from build123d import *

# Parameters (mm, degrees)
SKETCH1_R            = 30
BOSS_EXTRUDE1_DEPTH  = 75
SKETCH2_W            = 10
SKETCH2_H            = 56.81
SKETCH2_H_2          = 73.19
SKETCH3_R            = 3.175
BOSS_EXTRUDE2_DEPTH  = 10
SKETCH5_W            = 10
SKETCH5_H            = 20
CUT_EXTRUDE2_DEPTH   = 30
FILLET1_R            = 15
FILLET1_OF_MIRROR1_R = 15


with BuildPart() as part:
    # Sketch1 → Boss-Extrude1 (new, symmetric)
    with BuildSketch(Plane(origin=(0, 0, 0), x_dir=(1, 0, 0), z_dir=(0, 1, 0))):
        with Locations(Location((0, 0, 0), (0, 0, 270))):
            Circle(SKETCH1_R)
    extrude(amount=BOSS_EXTRUDE1_DEPTH, both=True)

    # Sketch2 → Cut-Revolve1 (revolve, cut)
    with BuildSketch(Plane(origin=(0, 0, 0), x_dir=(0, 0, -1), z_dir=(1, 0, 0))):
        with Locations((25, 36.595)):
            Rectangle(SKETCH2_W, SKETCH2_H)
        with Locations((25, -38.405)):
            Rectangle(SKETCH2_W, SKETCH2_H_2)
    revolve(axis=Axis((0, -1000, 0), (0, 1, 0)), mode=Mode.SUBTRACT)

    # Sketch3 → Boss-Extrude2 (add, symmetric)
    with BuildSketch(Plane(origin=(0, 0, 0), x_dir=(0, 0, -1), z_dir=(1, 0, 0))):
        Polygon((0, 75), (0, 60), (70, 60), (70, 85), (50, 85), (50, 75), align=None)
        with Locations((60, 75)):
            Circle(SKETCH3_R, mode=Mode.SUBTRACT)
    boss_extrude2 = extrude(amount=BOSS_EXTRUDE2_DEPTH, both=True)

    # Sketch5 → Cut-Extrude2 (cut)
    with BuildSketch(Plane(origin=(0, 0, -70), x_dir=(-1, 0, 0), z_dir=(0, 0, -1))):
        with Locations((0, 75)):
            Rectangle(SKETCH5_W, SKETCH5_H)
    cut_extrude2 = extrude(amount=-CUT_EXTRUDE2_DEPTH, mode=Mode.SUBTRACT)

    # Fillet1
    # the kernel refuses this fillet: 15 mm, written as the material it takes off along each edge
    with BuildSketch(Plane(origin=(-47.5, 60, -70), x_dir=(0, 0, 1), z_dir=(1, 0, 0))) as fillet1_piece_1:
        with BuildLine():
            CenterArc((FILLET1_R, -FILLET1_R), FILLET1_R, 90, 90)
            Line((0, -FILLET1_R), (0, 0))
            Line((0, 0), (FILLET1_R, 0))
        make_face()
    extrude(amount=95, mode=Mode.SUBTRACT)

    # Mirror1: Boss-Extrude2, Cut-Extrude2 across plane
    add(boss_extrude2.mirror(Plane.XY))
    add(cut_extrude2.mirror(Plane.XY), mode=Mode.SUBTRACT)

    # Fillet1 of Mirror1
    # the kernel refuses this fillet: 15 mm, written as the material it takes off along each edge
    with BuildSketch(Plane(origin=(-47.5, 60, 70), x_dir=(0, 0, -1), z_dir=(1, 0, 0))) as fillet1_of_mirror1_piece_1:
        with BuildLine():
            CenterArc((FILLET1_OF_MIRROR1_R, FILLET1_OF_MIRROR1_R), FILLET1_OF_MIRROR1_R, 180, 90)
            Line((0, FILLET1_OF_MIRROR1_R), (0, 0))
            Line((0, 0), (FILLET1_OF_MIRROR1_R, 0))
        make_face()
    extrude(amount=95, mode=Mode.SUBTRACT)


solid = part.part
Here's how the part is built. I have some questions about the finished solid (model axes, mm). A direction names the side the tool comes from. Round coordinates to 2 decimals unless told otherwise and drop trailing zeros. Order: outer loops, then holes, each group sorted by start corner. A loop starts at its lowest first (then second) coordinate and runs counter-clockwise, first axis right, second up. Notation, with made-up numbers: M -27.5,-24.75 L 14.5,-24.75 A25 cw 14.5,-11.75 Z; hole C 83,31.5 d7. An arc over 180 degrees is marked long. One line per question, with ' | ' between items.
1) I'm going to push flat-ended pins straight in: pin 1 Ø7.5 at (y, z) = (75, 60) entering from +X; pin 2 Ø18 at (x, z) = (-2, -1.5) entering from +Y; pin 3 Ø7.5 at (y, z) = (72, -36) entering from -X. Where does each tip first touch, or does it pass through?
Checked values:
pin 1: stops at x = 10 | pin 2: stops at y = 75 | pin 3: stops at x = -10
2) Imagine slicing it at A-A, the plane x = 0. Write out the boundary of the cut face in (y, z), plus the area to 3 significant figures.
Checked values:
outline: M -75,-20 L -1.81,-20 L -1.81,-30 L 8.19,-30 L 8.19,-20 L 60,-20 L 60,-55 A15 ccw 65,-66.18 L 65,-40 L 75,-40 L 75,40 L 65,40 L 65,66.18 A15 ccw 60,55 L 60,20 L 8.19,20 L 8.19,30 L -1.81,30 L -1.81,20 L -75,20 Z | area: 7,030 mm²
3) On a 3-axis mill with a long thin cutter (end or side, diameter ignored), from which of +Z, -Z, +X, -X, +Y, -Y can I reach the whole of each face in a straight line? I mean faces 4 (the flat face through (0, 75, -1)), 5 (the cylindrical face through (-7.535, 77.677, 61.707)), 6 (the flat face through (-5, 75, -55)), 7 (the flat face through (22, 65, 0)), 8 (the flat face through (20, 8.19, 6)). Say none if no direction works.
Checked values:
face 4: +X, -X, +Y | face 5: +X, -X | face 6: -Z, +Y | face 7: +X | face 8: none
4) Imagine slicing it at D-D, the plane z = -60. Write out the boundary of the cut face in (x, y) (3 decimals), plus the area to 3 significant figures.
Checked values:
outline: M -10,60.858 L 10,60.858 L 10,71.825 L 5,71.825 L 5,65 L -5,65 L -5,71.825 L -10,71.825 Z; M -10,78.175 L -5,78.175 L -5,85 L -10,85 Z; M 5,78.175 L 10,78.175 L 10,85 L 5,85 Z | area: 219 mm²
5) We'd pull the mould along X, two halves only. Please class faces 1 (the flat face through (5, 75, 55)), 2 (the cylindrical face through (19.524, -37.893, 4.336)), 3 (the cylindrical face through (29.996, 70.07, 0.517)): released by +X, released by -X, zero draft, split by the parting line, or undercut.
Checked values:
face 1: undercut | face 2: split by the parting line | face 3: released by +X
6) Imagine slicing it at B-B, the plane z = 0. Write out the boundary of the cut face in (x, y), plus the area to 3 significant figures.
Checked values:
outline: M -30,-1.81 L -20,-1.81 L -20,-75 L 20,-75 L 20,-1.81 L 30,-1.81 L 30,8.19 L 20,8.19 L 20,65 L 30,65 L 30,75 L -30,75 L -30,65 L -20,65 L -20,8.19 L -30,8.19 Z | area: 6,400 mm²
7) I need wall thicknesses on line 1 (Y direction, x = -6.5, z = 28); line 2 (Y direction, x = 23, z = -4); line 3 (Y direction, x = 7, z = 6). Which ranges of each line are inside material? Lowest first, please.
Checked values:
line 1: y = -1.81 to 8.19, 60 to 75 | line 2: y = -1.81 to 8.19, 65 to 75 | line 3: y = -75 to 75
8) Imagine slicing it at C-C, the plane y = -7. Write out the boundary of the cut face in (x, z).
Checked values:
outline: C 0,0 d40
